from build123d import *

# Parameters (mm, degrees)
SKETCH_1_R          = 1
EXTRUDE_1_DEPTH     = 3
FILLET_2_R          = 0.508
FILLET_3_R          = 1.27
SKETCH_3_W          = 2.895
SKETCH_3_H          = 3
CUT_EXTRUDE_1_DEPTH = 3


with BuildPart() as part:
    # 스케치1 → 보스-돌출1 (new body)
    with BuildSketch(Plane.XY):
        with BuildLine():
            ThreePointArc((-17.404694621, 2.689152768), (-14.003146094, 9.533383958), (-7.898975086, 14.132637079))
            ThreePointArc((-7.898975086, 14.132637079), (-3.181334345, 15.718511975), (1.784123639, 16.058159386))
            ThreePointArc((1.784123639, 16.058159386), (7.503730287, 15.09544823), (11.636286652, 11.025719632))
            ThreePointArc((11.636286652, 11.025719632), (12.626023912, 9.630255586), (13.939804575, 8.534408829))
            ThreePointArc((13.939804575, 8.534408829), (14.323714016, 7.94412001), (14.129144933, 7.267385039))
            ThreePointArc((14.129144933, 7.267385039), (12.117054941, 4.680354007), (11.583823092, 1.44664105))
            ThreePointArc((11.583823092, 1.44664105), (14.643044666, -3.801243579), (8.56860409, -3.783882772))
            ThreePointArc((8.56860409, -3.783882772), (4.032207962, -5.42180917), (1.784123639, -9.688870172))
            ThreePointArc((1.784123639, -9.688870172), (0, -16.2), (-1.784123639, -9.688870172))
            ThreePointArc((-1.784123639, -9.688870172), (-4.704806794, -5.722399103), (-9.262378909, -3.853758086))
            ThreePointArc((-9.262378909, -3.853758086), (-13.309581542, -6.642419158), (-16.154715264, -2.634714849))
            ThreePointArc((-16.154715264, -2.634714849), (-16.251667385, 0.151195755), (-17.404694621, 2.689152768))
        make_face()
        with Locations((-12.7, -3.195912181)):
            Circle(SKETCH_1_R, mode=Mode.SUBTRACT)
        with Locations((0, -12.7)):
            Circle(SKETCH_1_R, mode=Mode.SUBTRACT)
        with Locations((11.610795337, -2.05325502)):
            Circle(SKETCH_1_R, mode=Mode.SUBTRACT)
    extrude(amount=EXTRUDE_1_DEPTH)

    # 필렛2
    fillet_2_edges = [part.edges().sort_by_distance(p)[0] for p in [
        (14.129144933, 7.267385039, 1.5),
    ]]
    fillet(fillet_2_edges, radius=FILLET_2_R)

    # 필렛3
    fillet_3_edges = [part.edges().sort_by_distance(p)[0] for p in [
        (1.784123639, -9.688870172, 1.5),
        (-1.784123639, -9.688870172, 1.5),
        (-9.262378909, -3.853758086, 1.5),
        (-17.404694621, 2.689152768, 1.5),
        (11.583823092, 1.44664105, 1.5),
        (8.56860409, -3.783882772, 1.5),
    ]]
    fillet(fillet_3_edges, radius=FILLET_3_R)

    # 스케치3 → 컷-돌출1 (cut)
    with BuildSketch(Plane.XY.offset(3)):
        Polygon((-13.722156846, 6.885379209), (-11.210602391, 8.325212263), (-12.702657369, 10.927859366), (-15.214211823, 9.488026313), align=None)
        Polygon((-7.745048824, 11.302508101), (-4.968377523, 12.121728149), (-5.817310215, 14.999107735), (-8.593981516, 14.179887687), align=None)
        with Locations((2.188643344, 14.650807918)):
            Rectangle(SKETCH_3_W, SKETCH_3_H)
        Polygon((7.553748194, 11.804988601), (10.396441684, 11.257157677), (10.964142123, 14.20295404), (8.121448633, 14.750784964), align=None)
    extrude(amount=-CUT_EXTRUDE_1_DEPTH, mode=Mode.SUBTRACT)


solid = part.part
Geometry check sheet. Reference: the model listing, model coordinates, mm. A direction names the side the tool comes from. Round coordinates to 2 decimals unless told otherwise and drop trailing zeros. Order: outer loops, then holes, each group sorted by start corner. A loop starts at its lowest first (then second) coordinate and runs counter-clockwise, first axis right, second up. Notation, with made-up numbers: M 3.5,87.25 L 57.5,87.25 A30 ccw 57.5,116.25 Z; hole C 69.25,-24 d1. An arc over 180 degrees is marked long. Answer in a Markdown table with one row per item.
(1) Go/stop test with flat-tipped pins: P1, Ø1.6, axis at x = 11.61, y = -2.05, coming from the -Z side (3 decimals); P2, Ø0.9, axis at y = 15.5, z = 2, coming from the +X side. Record where each tip stops, or that it passes through.
Responses:
| item | result |
|---|---|
| P1 | passes through |
| P2 | stops at x = 7.59 |
(2) Sectioned sample at C-C, the plane z = 0.45. State how many separate pieces and enclosed holes the cut face has, and give its area (3 significant figures).
Responses:
| item | result |
|---|---|
| separate pieces | 1 |
| enclosed holes | 3 |
| area | 587 mm² |
(3) Draft check along Y on faces 1 (the face through (12.394, 5.24, 1.479)), 2 (the face through (-1, 4, 0)), 3 (the face through (-6.4, 11.7, 1.5)), 4 (the face through (2, 13.151, 2)). Enter one of: released by +Y, released by -Y, zero draft, split by the parting line, or undercut.
Responses:
| item | result |
|---|---|
| face 1 | undercut |
| face 2 | zero draft |
| face 3 | undercut |
| face 4 | released by +Y |
(4) Sectioned sample at D-D, the plane x = -4. Record the cut outline in (y, z), and give its area (3 significant figures).
Responses:
| item | result |
|---|---|
| outline | M -6.33,0 L 15.54,0 L 15.54,3 L -6.33,3 Z |
| area | 65.6 mm² |
(5) Scan lines: probe 1 along X at (y, z) = (-5, 1.8); probe 2 along X at (y, z) = (-2.5, 0.35); probe 3 along X at (y, z) = (-13, 2.8). Record each from-to range of solid material in increasing order. Write a range as from..to.
Responses:
| item | result |
|---|---|
| probe 1 | x = -15.7..-9.7, -5.78..4.57, 9.72..13.5 |
| probe 2 | x = -16.13..-13.42, -11.98..10.72, 12.51..15.08 |
| probe 3 | x = -3.49..-0.95, 0.95..3.49 |
(6) Tool access check on faces 5 (the face through (12.61, 9.65, 1.48)), 6 (the face through (10.52, 11.89, 1.52)), 7 (the face through (-5.387, 13.54, 1.521)). Record the directions out of +Z, -Z, +X, -X, +Y, -Y that give a thin tool (end or side, any length) a straight path to the whole face; none if there is none.
Responses:
| item | result |
|---|---|
| face 5 | +Z, -Z, +X, +Y |
| face 6 | +Z, -Z, +Y |
| face 7 | +Z, -Z |
(7) Sectioned sample at B-B, the plane x = 0. Record the cut outline in (y, z).
Responses:
| item | result |
|---|---|
| outline | M -16.2,0 L -13.7,0 L -13.7,3 L -16.2,3 Z; M -11.7,0 L 16.08,0 L 16.08,3 L -11.7,3 Z |
(8) Sectioned sample at A-A, the plane y = -12.7. Record the cut outline in (x, z), and give its area (3 significant figures).
Responses:
| item | result |
|---|---|
| outline | M -3.5,0 L -1,0 L -1,3 L -3.5,3 Z; M 1,0 L 3.5,0 L 3.5,3 L 1,3 Z |
| area | 15.0 mm² |
